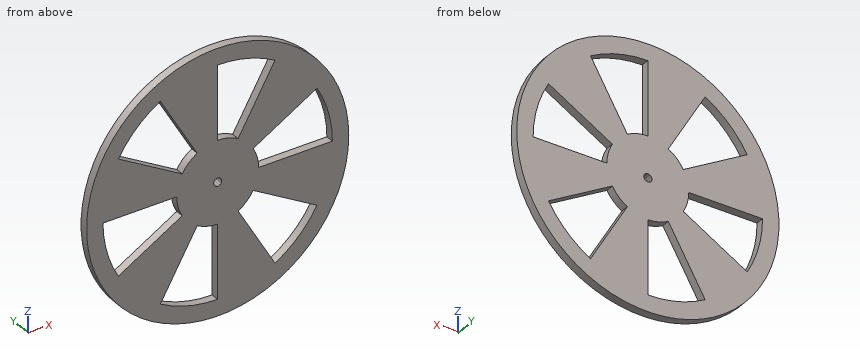
from build123d import *

# Parameters (mm, degrees)
F0_R     = 50.8
F1_DEPTH = 3.175


with BuildPart() as f1:
    # F0 (on Front) → F1 (new body)
    with BuildSketch(Plane.XZ):
        Circle(F0_R)
        with BuildLine():
            ThreePointArc((-38.494829, 22.225), (-31.430896, 31.430896), (-22.225, 38.494829))
            Line((-22.225, 38.494829), (-7.9375, 13.748153))
            ThreePointArc((-7.9375, 13.748153), (-4.108752, 15.334072), (0, 15.875))
            Line((0, 15.875), (0, 44.45))
            ThreePointArc((0, 44.45), (11.504507, 42.935403), (22.225, 38.494829))
            Line((22.225, 38.494829), (7.9375, 13.748153))
            ThreePointArc((7.9375, 13.748153), (11.22532, 11.22532), (13.748153, 7.9375))
            Line((13.748153, 7.9375), (38.494829, 22.225))
            ThreePointArc((38.494829, 22.225), (42.935403, 11.504507), (44.45, 0))
            Line((44.45, 0), (15.875, 0))
            ThreePointArc((15.875, 0), (15.334072, -4.108752), (13.748153, -7.9375))
            Line((13.748153, -7.9375), (38.494829, -22.225))
            ThreePointArc((38.494829, -22.225), (31.430896, -31.430896), (22.225, -38.494829))
            Line((22.225, -38.494829), (7.9375, -13.748153))
            ThreePointArc((7.9375, -13.748153), (4.108752, -15.334072), (0, -15.875))
            Line((0, -15.875), (0, -44.45))
            ThreePointArc((0, -44.45), (-11.504507, -42.935403), (-22.225, -38.494829))
            Line((-22.225, -38.494829), (-7.9375, -13.748153))
            ThreePointArc((-7.9375, -13.748153), (-11.22532, -11.22532), (-13.748153, -7.9375))
            Line((-13.748153, -7.9375), (-38.494829, -22.225))
            ThreePointArc((-38.494829, -22.225), (-42.935403, -11.504507), (-44.45, 0))
            Line((-44.45, 0), (-15.875, 0))
            ThreePointArc((-15.875, 0), (-15.334072, 4.108752), (-13.748153, 7.9375))
            Line((-13.748153, 7.9375), (-38.494829, 22.225))
        make_face(mode=Mode.SUBTRACT)
        with BuildLine():
            ThreePointArc((0, 15.875), (-4.108752, 15.334072), (-7.9375, 13.748153))
            ThreePointArc((-7.9375, 13.748153), (-11.22532, 11.22532), (-13.748153, 7.9375))
            ThreePointArc((-13.748153, 7.9375), (-15.334072, 4.108752), (-15.875, 0))
            ThreePointArc((-15.875, 0), (-15.334072, -4.108752), (-13.748153, -7.9375))
            ThreePointArc((-13.748153, -7.9375), (-11.22532, -11.22532), (-7.9375, -13.748153))
            ThreePointArc((-7.9375, -13.748153), (-4.108752, -15.334072), (0, -15.875))
            ThreePointArc((0, -15.875), (4.108752, -15.334072), (7.9375, -13.748153))
            ThreePointArc((7.9375, -13.748153), (11.22532, -11.22532), (13.748153, -7.9375))
            ThreePointArc((13.748153, -7.9375), (15.334072, -4.108752), (15.875, 0))
            ThreePointArc((15.875, 0), (15.334072, 4.108752), (13.748153, 7.9375))
            ThreePointArc((13.748153, 7.9375), (11.22532, 11.22532), (7.9375, 13.748153))
            ThreePointArc((7.9375, 13.748153), (4.108752, 15.334072), (0, 15.875))
        make_face()
        with BuildLine():
            ThreePointArc((1.374815, 0.79375), (1.533407, 0.410875), (1.5875, 0))
            ThreePointArc((1.5875, 0), (1.533407, -0.410875), (1.374815, -0.79375))
            ThreePointArc((1.374815, -0.79375), (1.122532, -1.122532), (0.79375, -1.374815))
            ThreePointArc((0.79375, -1.374815), (0.410875, -1.533407), (0, -1.5875))
            ThreePointArc((0, -1.5875), (-0.410875, -1.533407), (-0.79375, -1.374815))
            ThreePointArc((-0.79375, -1.374815), (-1.122532, -1.122532), (-1.374815, -0.79375))
            ThreePointArc((-1.374815, -0.79375), (-1.533407, -0.410875), (-1.5875, 0))
            ThreePointArc((-1.5875, 0), (-1.533407, 0.410875), (-1.374815, 0.79375))
            ThreePointArc((-1.374815, 0.79375), (-1.122532, 1.122532), (-0.79375, 1.374815))
            ThreePointArc((-0.79375, 1.374815), (-0.410875, 1.533407), (0, 1.5875))
            ThreePointArc((0, 1.5875), (0.410875, 1.533407), (0.79375, 1.374815))
            ThreePointArc((0.79375, 1.374815), (1.122532, 1.122532), (1.374815, 0.79375))
        make_face(mode=Mode.SUBTRACT)
    extrude(amount=F1_DEPTH)


solid = f1.part
Input: part model. Units: mm. Frame: model coordinates. Coordinates: 2 decimals unless noted, no trailing zeros. Order: outer loops, then holes, each group sorted by start corner. A loop starts at its lowest first (then second) coordinate and runs counter-clockwise, first axis right, second up. Notation, with made-up numbers: M 51,9 L 76,9 A13 cw 76,17 Z; hole C -16.5,-1 d11. An arc over 180 degrees is marked long. Write item = value, one per line. Start each with the question number.
(1) Section B-B on x = 4. Output: boundary loops of the cut face in (y, z) (3 decimals).
(2) Section A-A on z = -41. Output: boundary loops of the cut face in (x, y) (3 decimals), and give its area (3 significant figures).
(3) Section D-D on x = -19. Output: boundary loops of the cut face in (y, z) (3 decimals), and give its area (3 significant figures).
(4) First-contact query: P1, Ø1, axis at x = 34.5, y = -1.5, coming from the +Z side. Flat tip, straight axial feed; report the tip coordinate or a pass-through.
(5) Line query: line 1 along X through (y, z) = (-2.25, 10); line 2 along X through (y, z) = (-2.9, -30.5) (3 decimals); line 3 along Z through (x, y) = (-25, -2.7). Output: solid intervals per line, ascending. Write a range as [from, to].
(6) Section C-C on x = -32. Output: boundary loops of the cut face in (y, z) (3 decimals), and give its area (3 significant figures).
Result set:
q1.outline = M -3.175,-50.642 L 0,-50.642 L 0,15.363 L -3.175,15.363 Z; M -3.175,44.27 L 0,44.27 L 0,50.642 L -3.175,50.642 Z
q2.outline = M -29.994,-3.175 L -17.17,-3.175 L -17.17,0 L -29.994,0 Z; M 0,-3.175 L 29.994,-3.175 L 29.994,0 L 0,0 Z
q2.area = 136 mm²
q3.outline = M -3.175,-47.113 L 0,-47.113 L 0,-40.185 L -3.175,-40.185 Z; M -3.175,-32.909 L 0,-32.909 L 0,-10.97 L -3.175,-10.97 Z; M -3.175,0 L 0,0 L 0,10.97 L -3.175,10.97 Z; M -3.175,32.909 L 0,32.909 L 0,47.113 L -3.175,47.113 Z
q3.area = 172 mm²
q4.P1 = 37.74
q5.line_1 = [-49.81, -17.32], [-12.33, 17.32], [43.31, 49.81]
q5.line_2 = [-40.625, -17.609], [0, 17.609], [32.335, 40.625]
q5.line_3 = [-44.22, -14.43], [0, 14.43], [36.75, 44.22]
q6.outline = M -3.175,-39.454 L 0,-39.454 L 0,-18.475 L -3.175,-18.475 Z; M -3.175,0 L 0,0 L 0,18.475 L -3.175,18.475 Z; M -3.175,30.851 L 0,30.851 L 0,39.454 L -3.175,39.454 Z
q6.area = 153 mm²
